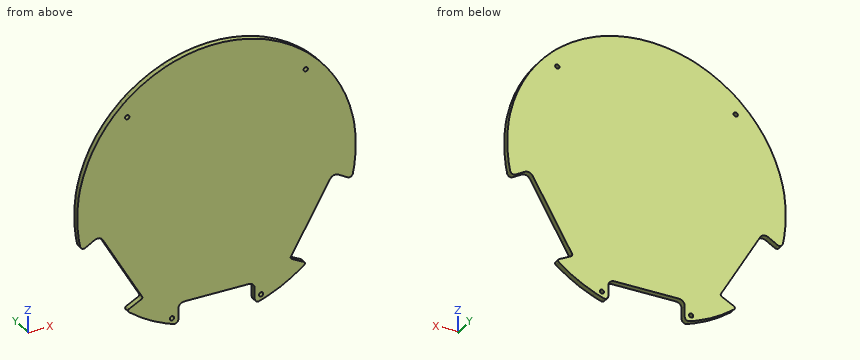
```python
from build123d import *

# Parameters (mm, degrees)
SKETCH1_R           = 1.15
BOSS_EXTRUDE2_DEPTH = 3


with BuildPart() as part:
    # Sketch1 → Boss-Extrude2 (new body)
    with BuildSketch(Plane(origin=(0, 0, 0), x_dir=(1, 0, 0), z_dir=(0, 1, 0))):
        with BuildLine():
            Line((17.353017405, 60.60705136), (-17.353017405, 60.60705136))
            ThreePointArc((-17.353017405, 60.60705136), (-19.629383429, 61.54995304), (-20.572285109, 63.826319064))
            Line((-20.572285109, 63.826319064), (-20.572285109, 69.573042322))
            ThreePointArc((-20.572285109, 69.573042322), (-21.350187318, 71.101515686), (-23.043737047, 71.372166724))
            ThreePointArc((-23.043737047, 71.372166724), (-25.323501925, 70.595469049), (-27.577152814, 69.745972233))
            ThreePointArc((-27.577152814, 69.745972233), (-37.5, 64.951905284), (-46.613207358, 58.755501017))
            ThreePointArc((-46.613207358, 58.755501017), (-46.906411899, 58.521692754), (-47.198443695, 58.286421342))
            ThreePointArc((-47.198443695, 58.286421342), (-47.564165172, 57.409734041), (-47.032034758, 56.622860452))
            Line((-47.032034758, 56.622860452), (-40.472942236, 53.197546407))
            ThreePointArc((-40.472942236, 53.197546407), (-39.975613978, 52.590341474), (-40.069820478, 51.811137802))
            Line((-40.069820478, 51.811137802), (-61.163754829, 15.275371775))
            ThreePointArc((-61.163754829, 15.275371775), (-63.118514649, 13.77543181), (-65.561356294, 14.097038013))
            Line((-65.561356294, 14.097038013), (-70.538164624, 16.970399642))
            ThreePointArc((-70.538164624, 16.970399642), (-72.250812491, 17.06095325), (-73.33197803, 15.729621681))
            ThreePointArc((-73.33197803, 15.729621681), (-73.799220551, 13.366938545), (-74.190360172, 10.990471215))
            ThreePointArc((-74.190360172, 10.990471215), (-75, 0), (-74.190360172, -10.990471215))
            ThreePointArc((-74.190360172, -10.990471215), (-73.794140163, -13.394957173), (-73.320012655, -15.785301525))
            ThreePointArc((-73.320012655, -15.785301525), (-64.937662855, -37.524657799), (-50.288240982, -55.642545043))
            ThreePointArc((-50.288240982, -55.642545043), (-48.475718626, -57.228530504), (-46.613207358, -58.755501017))
            ThreePointArc((-46.613207358, -58.755501017), (-37.5, -64.951905284), (-27.577152814, -69.745972233))
            ThreePointArc((-27.577152814, -69.745972233), (-25.296696887, -70.605078618), (-22.989534201, -71.389644328))
            ThreePointArc((-22.989534201, -71.389644328), (0.028475495, -74.999994594), (23.043737047, -71.372166724))
            ThreePointArc((23.043737047, -71.372166724), (25.323501925, -70.595469049), (27.577152814, -69.745972233))
            ThreePointArc((27.577152814, -69.745972233), (37.5, -64.951905284), (46.613207358, -58.755501017))
            ThreePointArc((46.613207358, -58.755501017), (48.497443275, -57.210121445), (50.330478454, -55.604342803))
            ThreePointArc((50.330478454, -55.604342803), (64.96613835, -37.475336795), (73.33197803, -15.729621681))
            ThreePointArc((73.33197803, -15.729621681), (73.799220551, -13.366938545), (74.190360172, -10.990471215))
            ThreePointArc((74.190360172, -10.990471215), (75, 0), (74.190360172, 10.990471215))
            ThreePointArc((74.190360172, 10.990471215), (73.799220551, 13.366938545), (73.33197803, 15.729621681))
            ThreePointArc((73.33197803, 15.729621681), (72.250812491, 17.06095325), (70.538164624, 16.970399642))
            Line((70.538164624, 16.970399642), (65.561356294, 14.097038013))
            ThreePointArc((65.561356294, 14.097038013), (63.118514649, 13.77543181), (61.163754829, 15.275371775))
            Line((61.163754829, 15.275371775), (43.810737424, 45.331679586))
            Line((43.810737424, 45.331679586), (40.069820478, 51.811137802))
            ThreePointArc((40.069820478, 51.811137802), (39.975613978, 52.590341474), (40.472942236, 53.197546407))
            Line((40.472942236, 53.197546407), (47.032034758, 56.622860452))
            ThreePointArc((47.032034758, 56.622860452), (47.564165172, 57.409734041), (47.198443695, 58.286421342))
            ThreePointArc((47.198443695, 58.286421342), (46.906411899, 58.521692754), (46.613207358, 58.755501017))
            ThreePointArc((46.613207358, 58.755501017), (37.5, 64.951905284), (27.577152814, 69.745972233))
            ThreePointArc((27.577152814, 69.745972233), (25.323501925, 70.595469049), (23.043737047, 71.372166724))
            ThreePointArc((23.043737047, 71.372166724), (21.350187318, 71.101515686), (20.572285109, 69.573042322))
            Line((20.572285109, 69.573042322), (20.572285109, 63.826319064))
            ThreePointArc((20.572285109, 63.826319064), (19.629383429, 61.54995304), (17.353017405, 60.60705136))
        make_face()
        with Locations(Location((-48, -48, 0), (0, 0, 270))):
            Circle(SKETCH1_R, mode=Mode.SUBTRACT)
        with Locations(Location((48, -48, 0), (0, 0, 270))):
            Circle(SKETCH1_R, mode=Mode.SUBTRACT)
        with Locations(Location((-24, 68, 0), (0, 0, 270))):
            Circle(SKETCH1_R, mode=Mode.SUBTRACT)
        with Locations(Location((24, 68, 0), (0, 0, 270))):
            Circle(SKETCH1_R, mode=Mode.SUBTRACT)
    extrude(amount=BOSS_EXTRUDE2_DEPTH)


solid = part.part
```
Check sheet for the modelled part. Datum: model origin and axes. Units: mm. Round coordinates to 2 decimals unless told otherwise and drop trailing zeros. Write each loop counter-clockwise with the first axis right and the second up, starting at its lowest first coordinate (ties: lowest second). Pieces come first, ordered by that corner, then holes. Notation, with made-up numbers: M -36,-16 L 21,-16 A20 cw 21,-2 Z; hole C 13.25,-3 d6. An arc over 180 degrees is marked long. Write item = value, one per line. Start each with the question number.
1. Scan lines: line 1 (X direction, y = 2.3, z = 48); line 2 (X direction, y = 1.6, z = -68); line 3 (X direction, y = 1.1, z = -40.5). Record each from-to range of solid material in increasing order. Write a range as [from, to].
2. Section check B-B, the plane x = 1.5. Record the cut outline in (y, z) (3 decimals), then the cut area to 3 significant figures.
3. Section check A-A, the plane y = 1.05. State how many separate pieces and enclosed holes the cut face has, then the cut area to 3 significant figures.
4. Section check C-C, the plane z = -49.5. Record the cut outline in (x, y).
5. Gauge pin test, flat ends, axial feed: pin 1 (1.5 mm diameter, centred on x = -5, y = 1.5, fed in from -Z); pin 2 (1.4 mm diameter, centred on x = -24, z = -68, fed in from -Y); pin 3 (1.5 mm diameter, centred on x = 45, y = 2.5, fed in from -Z); pin 4 (1 mm diameter, centred on y = 2.5, z = 37.5, fed in from +X). Record the tip position at first contact, or that the pin passes through.
Results found:
q1.line_1 = [-57.63, -49.15], [-46.85, 46.85], [49.15, 57.63]
q1.line_2 = [-31.64, -25.15], [-22.85, -20.57], [20.57, 22.85], [25.15, 31.64]
q1.line_3 = [-46.6, 46.6]
q2.outline = M 0,-60.607 L 3,-60.607 L 3,74.985 L 0,74.985 Z
q2.area = 407 mm^2
q3.separate_pieces = 1
q3.enclosed_holes = 4
q3.area = 15,900 mm^2
q4.outline = M -41.4,0 L 41.4,0 L 41.4,3 L -41.4,3 Z
q5.pin_1 = -60.61
q5.pin_2 = through
q5.pin_3 = -60.56
q5.pin_4 = 65.24
